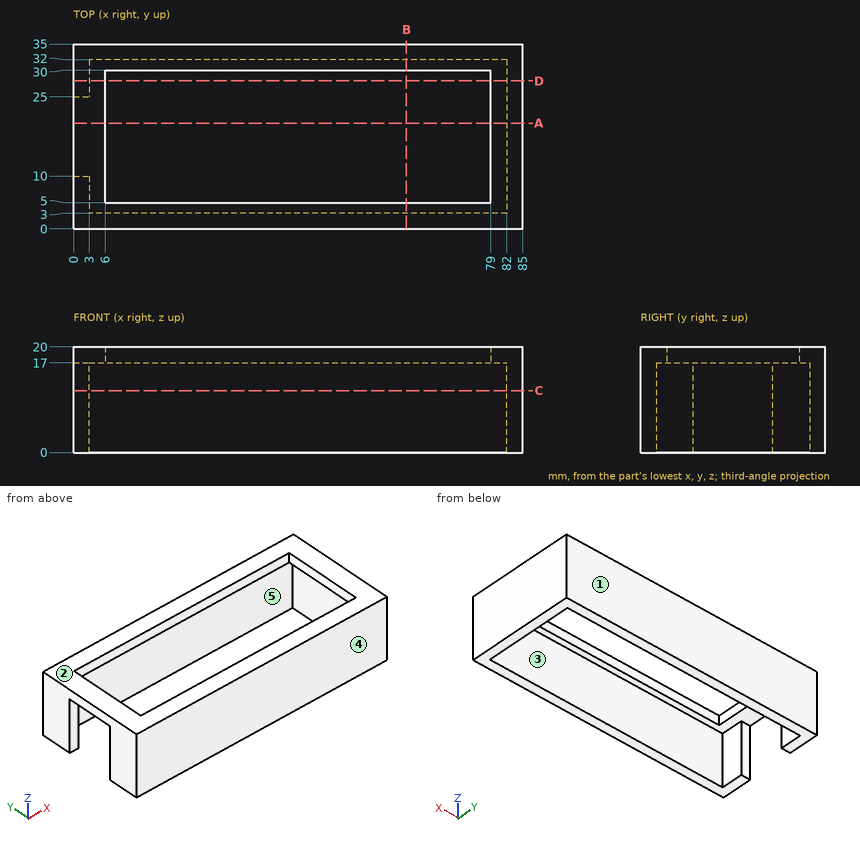
Check sheet for the drawn part. Datum: minimum x, y, z corner. Units: mm. A direction names the side the tool comes from. Coordinates: 2 decimals unless noted, no trailing zeros. Loops run counter-clockwise (first coordinate to the right, second up) from the corner with the lowest first, then second, coordinate; pieces in that order, holes last. Notation, with made-up numbers: (-27.5, 39.5) -> (13.5, 39.5) arc R18 ccw to (13.5, 48.5) -> close; hole circle Ø10 at (-19, 11.5). An arc over 180 degrees is marked (long way). Answer as a JSON object with one key per item and string values. Group by question number.
Item 1: Sectioned sample at C-C on z = 11.75. Record the boundary of the cut face in (x, y).
Item 2: Tool access check on the marked faces 4 and 5. Record the directions out of +Z, -Z, +X, -X, +Y, -Y that give a thin tool (end or side, any length) a straight path to the whole face; none if there is none.
Item 3: Scan lines: probe 1 along Y at (x, z) = (76.5, 5.25); probe 2 along X at (y, z) = (9, 12.5); probe 3 along Z at (x, y) = (38.5, 30.5). Record each from-to range of solid material in increasing order.
Item 4: Sectioned sample at B-B on x = 63. Record the boundary of the cut face in (y, z), plus the area to 3 significant figures.
Item 5: Sectioned sample at D-D on y = 28. Record the boundary of the cut face in (x, z), plus the area to 3 significant figures.
Item 6: Mould release check, pull along Y, two halves, no side actions. Record for the marked faces 1, 2 and 3: +Y half, -Y half, draft (parallel to the pull), parting line (faces both ways), or undercut.
Item 7: Sectioned sample at A-A on y = 20. Record the boundary of the cut face in (x, z), plus the area to 3 significant figures.
Item 8: Depth check by flat-ended pin: pin 1 (3 mm diameter, centred on y = 15.5, z = 11.5, fed in from -X). Enter the tip coordinate at first touch or a pass-through.
Evaluation:
{
 "1": {"outline": "(0, 0) -> (85, 0) -> (85, 35) -> (0, 35) -> (0, 25) -> (3, 25) -> (3, 32) -> (82, 32) -> (82, 3) -> (3, 3) -> (3, 10) -> (0, 10) -> close"},
 "2": {"face 4": "+Z, -Z, +X, -X, -Y", "face 5": "-Z"},
 "3": {"probe 1": "y = 0 to 3, 32 to 35", "probe 2": "x = 0 to 3, 82 to 85", "probe 3": "z = 17 to 20"},
 "4": {"outline": "(0, 0) -> (3, 0) -> (3, 17) -> (5, 17) -> (5, 20) -> (0, 20) -> close; (30, 17) -> (32, 17) -> (32, 0) -> (35, 0) -> (35, 20) -> (30, 20) -> close", "area": "132 mm²"},
 "5": {"outline": "(0, 0) -> (3, 0) -> (3, 17) -> (6, 17) -> (6, 20) -> (0, 20) -> close; (79, 17) -> (82, 17) -> (82, 0) -> (85, 0) -> (85, 20) -> (79, 20) -> close", "area": "138 mm²"},
 "6": {"face 1": "+Y half", "face 2": "draft", "face 3": "undercut"},
 "7": {"outline": "(0, 17) -> (6, 17) -> (6, 20) -> (0, 20) -> close; (79, 17) -> (82, 17) -> (82, 0) -> (85, 0) -> (85, 20) -> (79, 20) -> close", "area": "87.0 mm²"},
 "8": {"pin 1": "stops at x = 82"}
}
